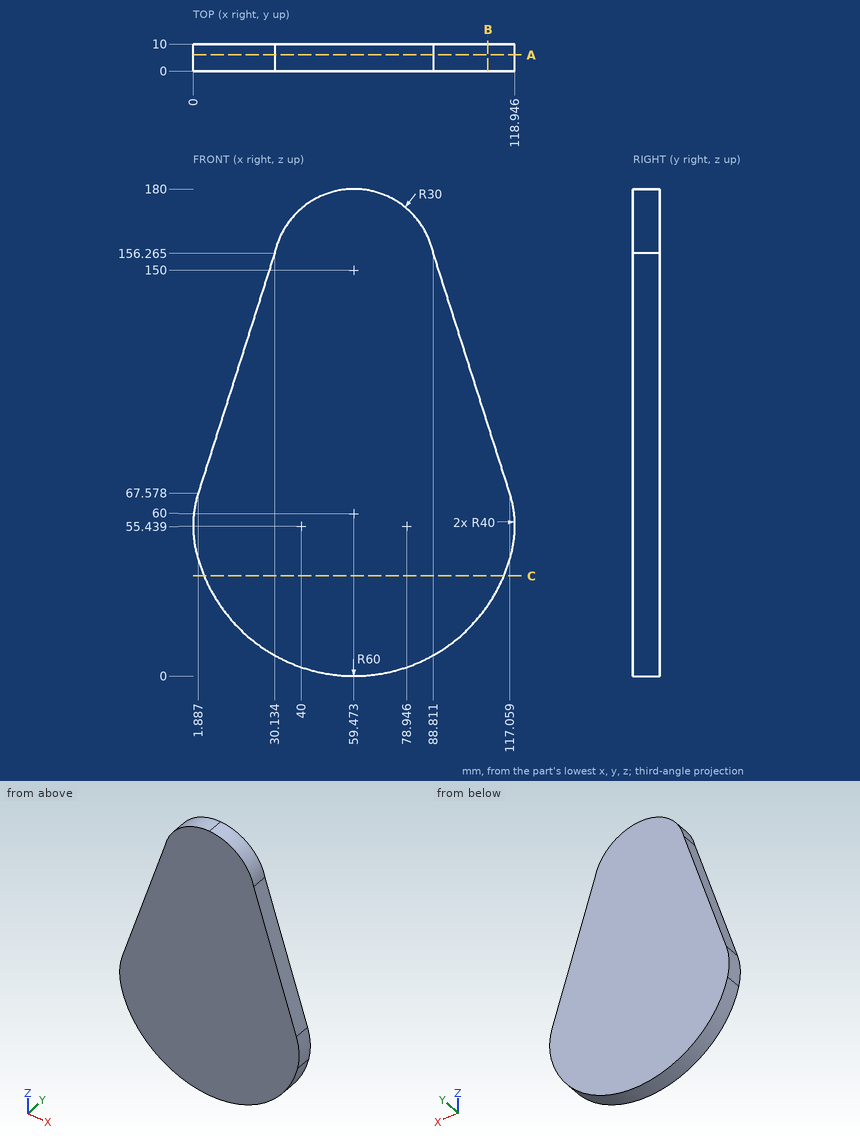
Input: dimensioned drawing with shaded views. Units: mm. Origin: part minimum x, y, z. Coordinates: 2 decimals unless noted, no trailing zeros. Write each loop counter-clockwise with the first axis right and the second up, starting at its lowest first coordinate (ties: lowest second). Pieces come first, ordered by that corner, then holes. Notation, with made-up numbers: M 68.5,32 L 82.5,32 A25 cw 82.5,60 Z; hole C 15.5,-22.5 d6. An arc over 180 degrees is marked long. Answer as a JSON object with one key per item and string values. Group by question number.
(1) Section A-A on y = 6. Output: boundary loops of the cut face in (x, z) (1 decimal), plus the area to 3 significant figures.
(2) Section C-C on z = 37. Output: boundary loops of the cut face in (x, y).
(3) Ray query, line 1 along X through (y, z) = (1.5, 132) (1 decimal); line 2 along X through (y, z) = (3, 169.5) (1 decimal); line 3 along Z through (x, y) = (46.5, 3.5). Return the intervals inside material, ascending. Write a range as [from, to].
(4) Contact query for flat-ended pins moving along their axis: P1, Ø1, axis at y = 3.5, z = 154.5, coming from the +X side; P2, Ø4, axis at x = 22.5, y = 1.5, coming from the -Z side (1 decimal); P3, Ø1, axis at y = 1.5, z = 121.5, coming from the -X side. Output: stop coordinate, or through.
(5) Section B-B on x = 109. Output: boundary loops of the cut face in (y, z).
Result set:
{
 "1": {"outline": "M 1.1,46.3 A60 ccw 117.9,46.3 A40 ccw 117.1,67.6 L 88.8,156.3 A30 ccw 59.5,180 A30 ccw 30.1,156.3 L 1.9,67.6 A40 ccw Z", "area": "15,300 mm2"},
 "2": {"outline": "M 4.06,0 L 114.89,0 L 114.89,10 L 4.06,10 Z"},
 "3": {"line 1": "x = [22.4, 96.5]", "line 2": "x = [36.7, 82.3]", "line 3": "z = [1.42, 177.05]"},
 "4": {"P1": "stops at x = 89.53", "P2": "stops at z = 11.2", "P3": "stops at x = 18.9"},
 "5": {"outline": "M 0,26.13 L 10,26.13 L 10,92.88 L 0,92.88 Z"}
}
